The listing builds one solid part. Answer for the finished solid, in the listing's coordinates (mm). Face numbers are marked on the shaded views. Round coordinates to 2 decimals unless told otherwise and drop trailing zeros. Order: outer loops, then holes, each group sorted by start corner. A loop starts at its lowest first (then second) coordinate and runs counter-clockwise, first axis right, second up. Notation, with made-up numbers: (84, 38) - (127, 38) arc R24 ccw to (127, 50) - close; hole circle Ø8 at (79, 78). An arc over 180 degrees is marked (long way). Write item = value, one per line.
from build123d import *

# Parameters (mm, degrees)
F0_R     = 3.175
F1_DEPTH = 76.2


with BuildPart() as f1:
    # F0 (on Front) → F1 (new body)
    with BuildSketch(Plane.XZ):
        with BuildLine():
            ThreePointArc((-69.372211, 40.419447), (-69.100298, 41.462677), (-69.008781, 42.53687))
            ThreePointArc((-69.008781, 42.53687), (-70.954579, 47.11131), (-75.599492, 48.882306))
            ThreePointArc((-75.599492, 48.882306), (-81.664762, 41.790478), (-74.111471, 36.310577))
            ThreePointArc((-74.111471, 36.310577), (-71.87486, 38.51844), (-69.372211, 40.419447))
        make_face()
        with Locations((-75.358781, 42.53687)):
            Circle(F0_R, mode=Mode.SUBTRACT)
        with BuildLine():
            ThreePointArc((-75.599492, 48.882306), (-70.954579, 47.11131), (-69.008781, 42.53687))
            ThreePointArc((-69.008781, 42.53687), (-69.100298, 41.462677), (-69.372211, 40.419447))
            ThreePointArc((-69.372211, 40.419447), (-56.911602, 44.443784), (-44.170318, 41.423559))
            ThreePointArc((-44.170318, 41.423559), (-58.546496, 50.792631), (-75.599492, 48.882306))
        make_face()
        with BuildLine():
            ThreePointArc((-74.111471, 36.310577), (-71.199098, 37.739001), (-69.372211, 40.419447))
            ThreePointArc((-69.372211, 40.419447), (-71.87486, 38.51844), (-74.111471, 36.310577))
        make_face()
    extrude(amount=F1_DEPTH)


solid = f1.part
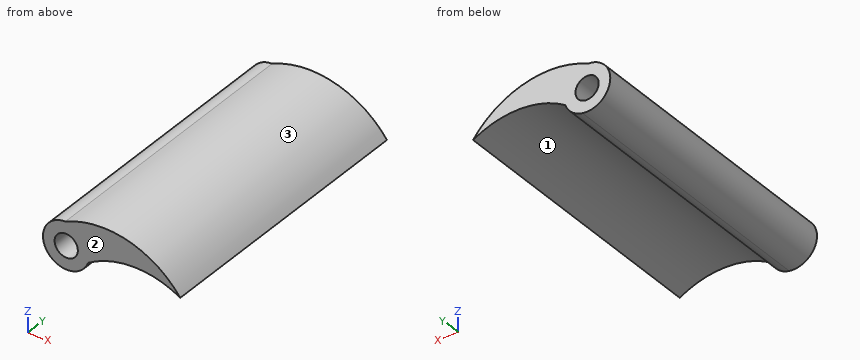
Q1. Section B-B on z = 38.5 is taken. Determine the outline of the cut face in (x, y), then the cut area to 3 significant figures.
Model answer:
outline = (-80.26, -76.2) - (-70.46, -76.2) - (-70.46, 0) - (-80.26, 0) - close
area = 747 mm^2
Q2. Determine the mould class of the marked faces 1, 2 and 3 for opening direction X: released by +X, released by -X, zero draft, split by the parting line, or undercut.
Model answer:
face_1 = undercut
face_2 = zero draft
face_3 = split by the parting line
Q3. Flat-ended cylindrical pins translate along their axes: P1, Ø3, axis at x = -66.5, y = -52.5, coming from the +Z side; P2, Ø1, axis at y = -19.5, z = 48.5, coming from the +X side; P3, Ø2, axis at x = -52.5, y = -33.5, coming from the -Z side. Find the tip coordinate at first contact, or state that the pin passes through.
Model answer:
P1 = 51.47
P2 = -51.58
P3 = 44.05
Q4. Find the intervals of material crossed by line 1 (X direction, y = -5, z = 45.25); line 2 (Z direction, x = -75, y = -46); line 3 (Z direction, x = -72.5, y = -59), in increasing order. Write a range as from..to.
Model answer:
line_1 = -81.1..-77.01, -73.71..-47.75
line_2 = 36.2..39.38, 45.69..49.17
line_3 = 36.87..41.16, 43.92..50.16
Q5. Section C-C on x = -54 is taken. Determine the outline of the cut face in (y, z), then the cut area to 3 significant figures.
Model answer:
outline = (-76.2, 44.39) - (0, 44.39) - (0, 49.25) - (-76.2, 49.25) - close
area = 370 mm^2
